```python
from build123d import *

# Parameters (mm, degrees)
F1_DEPTH    = 6.35
F2_T1_DEPTH = 38.1
F3_T1_DEPTH = 38.1
F5_R        = 3.17499
F6_R        = 3.175
F7_DEPTH    = 25.4


# Not quite as in the source:
# - a fillet or chamfer that OpenCascade refuses, or shapes differently, is made with other operations: its cross-section is extruded or revolved along the edge and cut away or added
# - a fillet or chamfer is up to 0.001 mm smaller than in the source, because OpenCascade refuses the exact size
# - a feature of the source that left no trace in its solid (it failed there, or was rolled back) is left out


with BuildPart() as f1:
    # F0 (on Front) → F1 (new body, symmetric)
    with BuildSketch(Plane.XZ):
        with BuildLine():
            Line((-81.1784485418, -7.2266137339), (-81.1784485418, 75.3233862661))
            Line((-81.1784485418, 75.3233862661), (-87.5284485418, 75.3233862661))
            Line((-87.5284485418, 75.3233862661), (-87.5284485418, -7.2266137339))
            ThreePointArc((-87.5284485418, -7.2266137339), (-80.0889607839, -25.1871259761), (-62.1284485418, -32.6266137339))
            Line((-62.1284485418, -32.6266137339), (2.9360103709, -32.6266137339))
            ThreePointArc((2.9360103709, -32.6266137339), (21.3157063883, -27.9002077014), (35.1353023462, -14.8936360074))
            Line((35.1353023462, -14.8936360074), (51.1881001208, 10.4850725552))
            Line((51.1881001208, 10.4850725552), (45.8215514582, 13.8795762674))
            Line((45.8215514582, 13.8795762674), (29.7687536837, -11.4991322951))
            ThreePointArc((29.7687536837, -11.4991322951), (18.2524237187, -22.3379420402), (2.9360103709, -26.2766137339))
            Line((2.9360103709, -26.2766137339), (-62.1284485418, -26.2766137339))
            ThreePointArc((-62.1284485418, -26.2766137339), (-75.5988327234, -20.6969979155), (-81.1784485418, -7.2266137339))
        make_face()
    extrude(amount=F1_DEPTH, both=True)

    # F2: fillet of radius 6.35 on 2 edges, made by hand

    # F2_s2 → F2_t1 (cut)
    with BuildSketch(Plane.YZ.offset(-103.4034485418)):
        with BuildLine():
            ThreePointArc((0, 75.3233862661), (4.4901280605, 73.4635143266), (6.35, 68.9733862661))
            Line((6.35, 68.9733862661), (6.35, 75.3233862661))
            Line((6.35, 75.3233862661), (0, 75.3233862661))
        make_face()
        with BuildLine():
            ThreePointArc((0, 75.3233862661), (-4.4901280605, 73.4635143266), (-6.35, 68.9733862661))
            Line((-6.35, 68.9733862661), (-6.35, 75.3233862661))
            Line((-6.35, 75.3233862661), (0, 75.3233862661))
        make_face()
    extrude(amount=F2_T1_DEPTH, mode=Mode.SUBTRACT)

    # F3: fillet of radius 6.35 on 2 edges, made by hand

    # F3_s2 → F3_t1 (cut)
    with BuildSketch(Plane(origin=(45.2399237114, 0, -28.6156147341), x_dir=(0, 1, 0), z_dir=(-0.8451257736, 0, 0.5345675137))):
        with BuildLine():
            ThreePointArc((-6.35, -29.8747004693), (-4.4901280605, -34.3648285299), (0, -36.2247004693))
            Line((0, -36.2247004693), (-6.35, -36.2247004693))
            Line((-6.35, -36.2247004693), (-6.35, -29.8747004693))
        make_face()
        with BuildLine():
            ThreePointArc((6.35, -29.8747004693), (4.4901280605, -34.3648285299), (0, -36.2247004693))
            Line((0, -36.2247004693), (6.35, -36.2247004693))
            Line((6.35, -36.2247004693), (6.35, -29.8747004693))
        make_face()
    extrude(amount=F3_T1_DEPTH, mode=Mode.SUBTRACT)

    # F5 (radius 3.175 in the source; OpenCascade refuses exactly that, so slightly less here)
    f5_edges = [f1.edges().sort_by_distance(p)[0] for p in [
        (-81.178449, -6.35, 30.873386),
        (18.252424, 6.35, -22.337942),
        (18.252424, -6.35, -22.337942),
        (41.464449, 6.35, -4.887556),
        (21.315706, 6.35, -27.900208),
        (-29.596219, 6.35, -32.626614),
        (-80.088961, 6.35, -25.187126),
        (-87.528449, 6.35, 30.873386),
        (-81.178449, 6.35, 30.873386),
        (-75.598833, 6.35, -20.696998),
        (-29.596219, 6.35, -26.276614),
        (36.097901, 6.35, -1.493052),
        (-29.596219, -6.35, -26.276614),
        (41.464449, -6.35, -4.887556),
        (21.315706, -6.35, -27.900208),
        (-29.596219, -6.35, -32.626614),
        (-80.088961, -6.35, -25.187126),
        (-87.528449, -6.35, 30.873386),
        (-75.598833, -6.35, -20.696998),
        (36.097901, -6.35, -1.493052),
        (44.827324, 4.490128, 12.307751),
        (44.827324, -4.490128, 12.307751),
        (50.193873, 4.490128, 8.913247),
        (50.193873, -4.490128, 8.913247),
        (-87.528449, -4.490128, 73.463514),
        (-87.528449, 4.490128, 73.463514),
        (-81.178449, 4.490128, 73.463514),
        (-81.178449, -4.490128, 73.463514),
    ]]
    fillet(f5_edges, radius=F5_R)

    # F6 (on face) → F7 (cut)
    with BuildSketch(Plane(origin=(-87.5284485418, 0, 0), x_dir=(0, -1, 0), z_dir=(-1, 0, 0))):
        with Locations((0, 65.7983862661)):
            Circle(F6_R)
        with Locations((0, 40.3983862661)):
            Circle(F6_R)
    extrude(amount=-F7_DEPTH, mode=Mode.SUBTRACT)


solid = f1.part
```
Work out the finished part from the listing and answer in its coordinate system (mm). A direction names the side the tool comes from. Give positions to 0.01 mm unless a question says otherwise; leave off trailing zeros. One line per question, with ' | ' between items.
(1) A tool of negligible diameter and unlimited length cuts with its end or side. For faces 1 (the face through (36.774, -5.395, -2.117)), 2 (the face through (36.952, 5.395, -1.837)), 3 (the face through (-29, 0, -26.277)), 4 (the face through (21.08, -0.04, -28.03)), from which of +Z, -Z, +X, -X, +Y, -Y can it reach the whole face along a straight path? Write none if from no direction.
Recorded:
face 1: +Z, -Y | face 2: +Z, +Y | face 3: +Z, +Y, -Y | face 4: -Z, +X, +Y, -Y
(2) Each of these flat-tipped pins is pushed along its axis until it touches: pin 1 Ø1.5 at (x, y) = (-22.5, 0.5) entering from +Z; pin 2 Ø5 at (y, z) = (0, 65.8) entering from -X; pin 3 Ø3 at (x, y) = (23.5, 1) entering from -Z; pin 4 Ø7 at (y, z) = (-1.5, 45) entering from +X. Where does it stop, or does it pass through?
Recorded:
pin 1: stops at z = -26.28 | pin 2: passes through | pin 3: stops at z = -27.51 | pin 4: stops at x = -81.18
(3) Straight lines are drawn through the part: probe 1 along X at (y, z) = (1, 62); probe 2 along X at (y, z) = (-1.5, -15); probe 3 along Z at (x, y) = (-59, 2). For each, find the intervals that lie inside material, in ascending order.
Recorded:
probe 1: x = -87.53 to -81.18 | probe 2: x = -86.31 to -79.52, 27.2 to 35.07 | probe 3: z = -32.63 to -26.28
(4) The mould has two halves that part along Z. Classify faces 5 (the face through (-75.45, -0.044, -20.844)), 6 (the face through (-29.141, 5.445, -31.672)), 7 (the face through (-84.398, 2.34, 67.944)): +Z half, -Z half, draft (parallel to the pull), parting line (faces both ways), or undercut.
Recorded:
face 5: +Z half | face 6: -Z half | face 7: undercut
